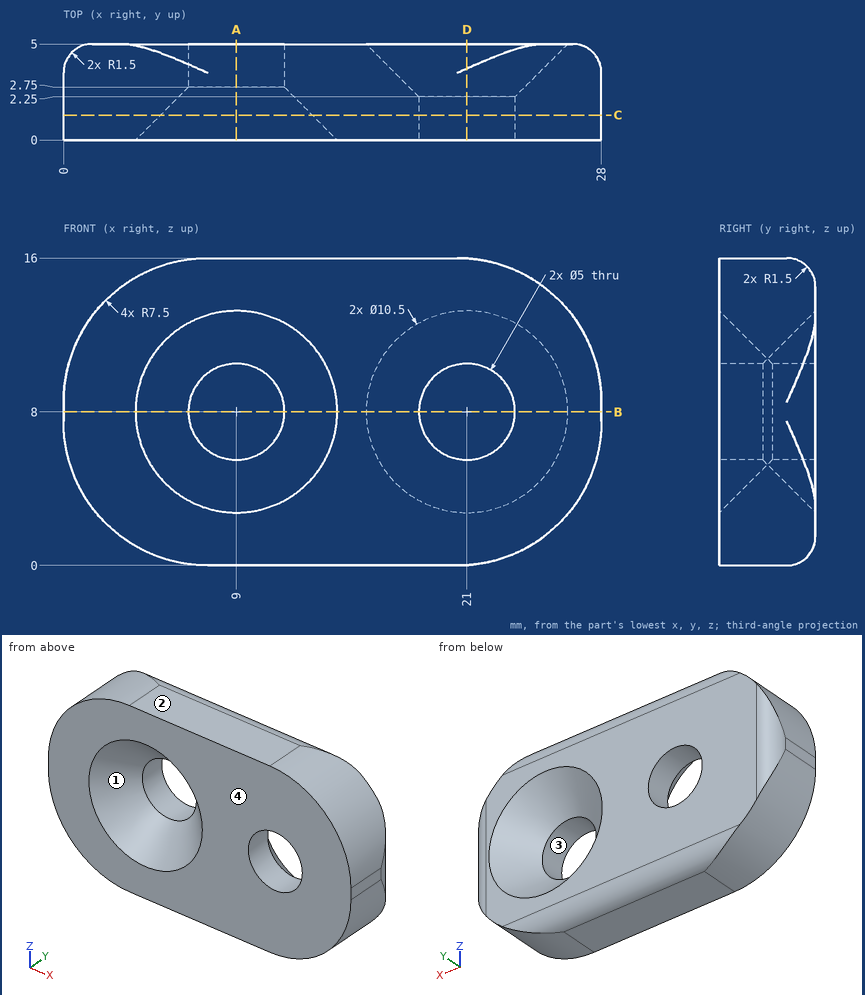
Geometry check sheet. Reference: drawing and pictorial views, mm from the part's lowest x, y, z. Give positions to 0.01 mm unless a question says otherwise; leave off trailing zeros. Write each loop counter-clockwise with the first axis right and the second up, starting at its lowest first coordinate (ties: lowest second). Pieces come first, ordered by that corner, then holes. Notation, with made-up numbers: (68, -24) -> (101, -24) arc R28 cw to (101, -5) -> close; hole circle Ø5 at (29, 10). An arc over 180 degrees is marked (long way). One line per item, written item: value. Start each with the question number.
Item 1: Section check A-A on x = 9. Record the cut outline in (y, z), then the cut area to 3 significant figures.
Item 2: Section check D-D on x = 21. Record the cut outline in (y, z).
Item 3: Section check C-C on y = 1.3. Record the cut outline in (x, z), then the cut area to 3 significant figures.
Item 4: Gauge pin test, flat ends, axial feed: pin 1 (1 mm diameter, centred on y = 4.5, z = 7.5, fed in from +X); pin 2 (1.5 mm diameter, centred on y = 2.5, z = 6.5, fed in from -X); pin 3 (1 mm diameter, centred on y = 2.5, z = 5.5, fed in from -X); pin 4 (4.5 mm diameter, centred on x = 9, z = 8, fed in from +Y). Record the tip position at first contact, or that the pin passes through.
Item 5: Section check B-B on z = 8. Record the cut outline in (x, y).
Item 6: Draft check along Z on the marked faces 1, 2, 3 and 4. Enter one of: +Z half, -Z half, draft (parallel to the pull), parting line (faces both ways), or undercut.
Item 7: Material ranges on probe 1 along X at (y, z) = (1.05, 13); probe 2 along Z at (x, y) = (21.75, 2.9); probe 3 along Z at (x, y) = (9.75, 0.6), recorded low to high. Write a range as from..to.
Results list:
1. outline: (0, 0) -> (3.5, 0) arc R1.5 ccw to (5, 1.5) -> (5, 5.5) -> (2.75, 5.5) -> (0, 2.75) -> close; (0, 13.25) -> (2.75, 10.5) -> (5, 10.5) -> (5, 14.5) arc R1.5 ccw to (3.5, 16) -> (0, 16) -> close
1. area: 46.5 mm²
2. outline: (0, 0.02) -> (3.72, 0.02) arc R1.5 ccw to (5, 1.5) -> (5, 2.75) -> (2.25, 5.5) -> (0, 5.5) -> close; (0, 10.5) -> (2.25, 10.5) -> (5, 13.25) -> (5, 14.5) arc R1.5 ccw to (3.72, 15.98) -> (0, 15.98) -> close
3. outline: (0, 7.5) arc R7.5 ccw to (7.5, 0) -> (20.5, 0) arc R7.5 ccw to (28, 7.5) -> (28, 8.5) arc R7.5 ccw to (20.5, 16) -> (7.5, 16) arc R7.5 ccw to (0, 8.5) -> close; hole circle Ø7.9 at (9, 8); hole circle Ø5 at (21, 8)
3. area: 331 mm²
4. pin 1: x = 27.91
4. pin 2: x = 0
4. pin 3: x = 0.15
4. pin 4: through
5. outline: (0, 0) -> (3.75, 0) -> (6.5, 2.75) -> (6.5, 5) -> (1.5, 5) arc R1.5 ccw to (0, 3.5) -> close; (11.5, 2.75) -> (14.25, 0) -> (18.5, 0) -> (18.5, 2.25) -> (15.75, 5) -> (11.5, 5) -> close; (23.5, 0) -> (28, 0) -> (28, 3.5) arc R1.5 ccw to (26.5, 5) -> (26.25, 5) -> (23.5, 2.25) -> close
6. face 1: undercut
6. face 2: +Z half
6. face 3: undercut
6. face 4: draft
7. probe 1: 1.5..26.5
7. probe 2: 0.1..4.94, 11.06..15.9
7. probe 3: 0..3.41, 12.59..16
